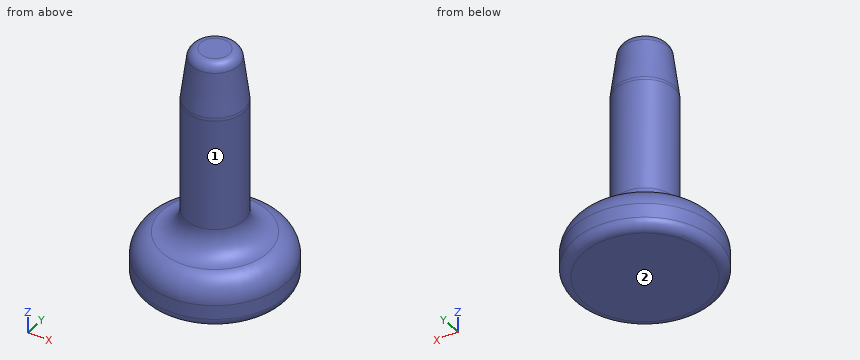
from build123d import *


with BuildPart() as f1:
    # F0 (on Front) → F1 (revolve)
    with BuildSketch(Plane.XZ):
        with BuildLine():
            Line((0, 0), (0, 50))
            Line((0, 50), (-2.988412, 50))
            ThreePointArc((-2.988412, 50), (-4.310339, 49.500836), (-4.972408, 48.252509))
            Line((-4.972408, 48.252509), (-6.10999, 39.314368))
            ThreePointArc((-6.10999, 39.314368), (-6.139987, 38.999365), (-6.15, 38.683096))
            Line((-6.15, 38.683096), (-6.15, 15))
            ThreePointArc((-6.15, 15), (-7.614466, 11.464466), (-11.15, 10))
            Line((-11.15, 10), (-10, 10))
            ThreePointArc((-10, 10), (-13.535534, 8.535534), (-15, 5))
            Line((-15, 5), (-15, 2))
            ThreePointArc((-15, 2), (-14.414214, 0.585786), (-13, 0))
            Line((-13, 0), (0, 0))
        make_face()
    revolve(axis=Axis((0, 0, 25), (0, 0, -1)))


solid = f1.part
Verification items for the finished model (mm, model axes). Face numbers are marked on the shaded views. A direction names the side the tool comes from. Give positions to 0.01 mm unless a question says otherwise; leave off trailing zeros. Order: outer loops, then holes, each group sorted by start corner. A loop starts at its lowest first (then second) coordinate and runs counter-clockwise, first axis right, second up. Notation, with made-up numbers: M -6,85.5 L 12,85.5 A32 ccw 12,119.5 Z; hole C 79.25,67.5 d5. An arc over 180 degrees is marked long. Use one line per item in the form item = value. Start each with the question number.
Q1. Access from +Z, -Z, +X, -X, +Y, -Y to the whole of each face (thin tool, end or side, straight path). Record for the marked faces 1 and 2.
Q2. Go/stop test with flat-tipped pins: pin 1 Ø1.5 at (y, z) = (5, 26) entering from -X; pin 2 Ø2 at (x, z) = (-4, 38) entering from +Y; pin 3 Ø2 at (x, y) = (11, -9) entering from -Z; pin 4 Ø10 at (y, z) = (11, 43.5) entering from -X. Record where each tip stops, or that it passes through.
Q3. Scan lines: line 1 along Y through (x, z) = (0, 35); line 2 along Z through (x, y) = (9.5, -6); line 3 along X through (y, z) = (-2, 19). Record each from-to range of solid material in increasing order. Write a range as [from, to].
Q4. Section check B-B (z = 29). Enter the section's corners in (x, y), then the cut area to 3 significant figures.
Q5. Section check A-A (z = 12). Enter the section's corners in (x, y), then the cut area to 3 significant figures.
Evaluation:
q1.face_1 = +Z
q1.face_2 = -Z, +X, -X, +Y, -Y
q2.pin_1 = -4.45
q2.pin_2 = 5.37
q2.pin_3 = 0.01
q2.pin_4 = through
q3.line_1 = [-6.15, 6.15]
q3.line_2 = [0, 9.84]
q3.line_3 = [-5.82, 5.82]
q4.outline = C 0,0 d12.3
q4.area = 119 mm2
q5.outline = C 0,0 d14.3
q5.area = 161 mm2
